The model under review builds one solid part; all positions refer to its coordinate system, in mm. A direction names the side the tool comes from. Coordinates: 2 decimals unless noted, no trailing zeros. Loops run counter-clockwise (first coordinate to the right, second up) from the corner with the lowest first, then second, coordinate; pieces in that order, holes last. Notation, with made-up numbers: M 26.5,34.5 L 83.5,34.5 A18 ccw 83.5,42.5 Z; hole C -37.75,-5 d6. An arc over 180 degrees is marked long. Write item = value, one per line. Start each with the question number.
Q1. Clearance check with flat-ended pins moving along their axes: pin 1 Ø4 at (y, z) = (46.5, 10.5) entering from +X; pin 2 Ø4 at (x, z) = (33.5, 3.5) entering from +Y; pin 3 Ø3.5 at (y, z) = (68, 9) entering from +X. State where each tip first meets the part, or that it passes through.
Q2. We need section B-B on z = 20. Give the boundary of the cut face in (x, y), and give its area (3 significant figures).
Q3. We need section D-D on x = 29.5. Give the boundary of the cut face in (y, z).
Q4. Wall thickness on probe 1 along Z at (x, y) = (-20, 68.5); probe 2 along Z at (x, y) = (-20.5, 67.5); probe 3 along Y at (x, z) = (2, 13.5): over which ranges is each line inside the solid? List them lowest first.
Q5. We need section C-C on y = 17. Give the boundary of the cut face in (x, z), and give its area (3 significant figures).
Q6. For faces 4 (the face through (-13, 63, 13)), 5 (the face through (0, 67, 12)), 6 (the face through (-5.8, 67.9, 6.5)), list the 3-axis set-ups (+Z, -Z, +X, -X, +Y, -Y) from which the entire face can be reached by the end or side of a thin tool; tool diameter is ignored.
Q7. We need section A-A on x = -20. Give the boundary of the cut face in (y, z), and give its area (3 significant figures).
Q8. Mouldability with a two-part tool opening along Y and no side actions: class faces 1 (the face through (71.406, -13.449, 11.036)), 2 (the face through (71.3, -21.9, 21.4)), 3 (the face through (-12, 73, 12)) as released by +Y, released by -Y, zero draft, split by the parting line, or undercut.
from build123d import *

# Parameters (mm, degrees)
BOSS_EXTRUDE1_DEPTH  = 25
CUT_EXTRUDE1_REACH   = 127.103
SKETCH6_R            = 1.5
FILLET1_R            = 12.5
SKETCH8_W            = 25
SKETCH8_H            = 25
BOSS_EXTRUDE2_DEPTH  = 7
FILLET2_R            = 2
M3_CLEARANCE_HOLE1_D = 3.4


with BuildPart() as part:
    # Sketch2 → Boss-Extrude1 (new body)
    with BuildSketch(Plane.XY):
        with BuildLine():
            Line((0, 73), (-25, 73))
            Line((-25, 73), (-25, 70))
            Line((-25, 70), (0, 70))
            ThreePointArc((0, 70), (49.712976294, 49.281030712), (69.997334614, -0.610857485))
            Line((69.997334614, -0.610857485), (69.779171227, -25.609905561))
            Line((69.779171227, -25.609905561), (72.779056996, -25.636085168))
            Line((72.779056996, -25.636085168), (72.997220384, -0.637037091))
            ThreePointArc((72.997220384, -0.637037091), (51.84353242, 51.393074885), (0, 73))
        make_face()
    extrude(amount=BOSS_EXTRUDE1_DEPTH)

    # Sketch6 → Cut-Extrude1 (cut, up to next)
    with BuildSketch(Plane(origin=(72.997220384, -0.637037091, 0), x_dir=(0, 0, -1), z_dir=(0.9999619230641714, -0.00872653549837746, 0)), mode=Mode.PRIVATE) as cut_extrude1_sk1:
        with Locations(Location((-12.5, -12.5, 0), (0, 0, 90))):
            Circle(SKETCH6_R)
    cut_extrude1_tool1 = extrude(cut_extrude1_sk1.sketch, amount=-CUT_EXTRUDE1_REACH, mode=Mode.PRIVATE) & part.part
    add(cut_extrude1_tool1.solids().sort_by_distance((72.888139, -13.136561, 12.5))[0], mode=Mode.SUBTRACT)

    # Fillet1
    fillet1_edges = [part.edges().sort_by_distance(p)[0] for p in [
        (71.279114112, -25.622995365, 0),
        (71.279114112, -25.622995365, 25),
    ]]
    fillet(fillet1_edges, radius=FILLET1_R - 0.0001)  # a hair under: the kernel refuses the full size

    # Sketch8 → Boss-Extrude2 (add)
    with BuildSketch(Plane.XZ.offset(-70)):
        with Locations((-12.5, 12.5)):
            Rectangle(SKETCH8_W, SKETCH8_H)
    extrude(amount=BOSS_EXTRUDE2_DEPTH)

    # Fillet2
    fillet2_edges = [part.edges().sort_by_distance(p)[0] for p in [
        (-25, 68, 25),
        (-25, 68, 0),
    ]]
    fillet(fillet2_edges, radius=FILLET2_R)

    # M3 Clearance Hole1 (through all)
    with Locations(Plane(origin=(0, 73, 0), x_dir=(1, 0, 0), z_dir=(0, 1, 0))):
        with Locations((-20, -5), (-5, -20), (-20, -20), (-5, -5)):
            Hole(M3_CLEARANCE_HOLE1_D / 2)


solid = part.part
Returned:
q1.pin_1 = 57.87
q1.pin_2 = 65.85
q1.pin_3 = 30.66
q2.outline = M -25,63 L -21.7,63 L -21.7,73 L -25,73 Z; M -18.3,63 L -6.7,63 L -6.7,73 L -18.3,73 Z; M -3.3,63 L 0,63 L 0,70 A70 cw 70,-0.61 L 69.8,-23.11 L 72.8,-23.14 L 73,-0.64 A73 ccw 0,73 L -3.3,73 Z
q2.area = 588 mm^2
q3.outline = M 63.48,0 L 66.77,0 L 66.77,25 L 63.48,25 Z
q4.probe_1 = 0 to 3.3, 6.7 to 18.3, 21.7 to 25
q4.probe_2 = 0 to 3.38, 6.62 to 18.38, 21.62 to 25
q4.probe_3 = 69.97 to 72.97
q5.outline = M 67.9,0 L 70.99,0 L 70.99,25 L 67.9,25 Z
q5.area = 77.2 mm^2
q6.face_4 = +Z, -Z, -X, -Y
q6.face_5 = +Z, -Z, -Y
q6.face_6 = +Y, -Y
q7.outline = M 63,0 L 73,0 L 73,3.3 L 63,3.3 Z; M 63,6.7 L 73,6.7 L 73,18.3 L 63,18.3 Z; M 63,21.7 L 73,21.7 L 73,25 L 63,25 Z
q7.area = 182 mm^2
q8.face_1 = undercut
q8.face_2 = released by -Y
q8.face_3 = released by +Y
